Source: CAD feature listing. Evaluate the final solid. Frame: model axes, mm. Face numbers are marked on the shaded views. A direction names the side the tool comes from. Coordinates: 2 decimals unless noted, no trailing zeros. Write each loop counter-clockwise with the first axis right and the second up, starting at its lowest first coordinate (ties: lowest second). Pieces come first, ordered by that corner, then holes. Notation, with made-up numbers: (-13, 0.5) - (46, 0.5) arc R16 cw to (46, 24.5) - close; hole circle Ø3 at (72.25, 85.5). An arc over 180 degrees is marked (long way). One line per item, written item: value.
from build123d import *

# Parameters (mm, degrees)
SKETCH1_R           = 42.5
SKETCH1_R_2         = 12
BOSS_EXTRUDE1_DEPTH = 5
SKETCH2_R           = 32.5
SKETCH2_R_2         = 6.5
BOSS_EXTRUDE2_DEPTH = 10
SKETCH3_R           = 4
BOSS_EXTRUDE3_DEPTH = 10
SKETCH5_R           = 2.5
CUT_EXTRUDE1_DEPTH  = 10
SKETCH7_R           = 2.5
CUT_EXTRUDE2_DEPTH  = 10


with BuildPart() as part:
    # Sketch1 → Boss-Extrude1 (new body)
    with BuildSketch(Plane.XY):
        Circle(SKETCH1_R)
        Circle(SKETCH1_R_2, mode=Mode.SUBTRACT)
    extrude(amount=BOSS_EXTRUDE1_DEPTH)

    # Sketch2 → Boss-Extrude2 (add)
    with BuildSketch(Plane.XY.offset(5)):
        Circle(SKETCH2_R)
        Circle(SKETCH2_R_2, mode=Mode.SUBTRACT)
    extrude(amount=BOSS_EXTRUDE2_DEPTH)

    # Sketch3 → Boss-Extrude3 (add)
    with BuildSketch(Plane(origin=(0, 0, 0), x_dir=(-1, 0, 0), z_dir=(0, 0, -1))):
        with Locations(Location((0, 22.5, 0), (0, 0, 180))):
            Circle(SKETCH3_R)
        with Locations(Location((15.909902577, 15.909902577, 0), (0, 0, 180))):
            Circle(SKETCH3_R)
        with Locations(Location((22.5, 0, 0), (0, 0, 180))):
            Circle(SKETCH3_R)
        with Locations(Location((15.909902577, -15.909902577, 0), (0, 0, 180))):
            Circle(SKETCH3_R)
        with Locations(Location((0, -22.5, 0), (0, 0, 180))):
            Circle(SKETCH3_R)
        with Locations(Location((-15.909902577, -15.909902577, 0), (0, 0, 180))):
            Circle(SKETCH3_R)
        with Locations(Location((-22.5, 0, 0), (0, 0, 180))):
            Circle(SKETCH3_R)
        with Locations(Location((-15.909902577, 15.909902577, 0), (0, 0, 180))):
            Circle(SKETCH3_R)
    extrude(amount=BOSS_EXTRUDE3_DEPTH)

    # Sketch5 → Cut-Extrude1 (cut)
    with BuildSketch(Plane.XY.offset(15)):
        with Locations((0, 25)):
            Circle(SKETCH5_R)
        with Locations((21.650635095, 12.5)):
            Circle(SKETCH5_R)
        with Locations((21.650635095, -12.5)):
            Circle(SKETCH5_R)
        with Locations((0, -25)):
            Circle(SKETCH5_R)
        with Locations((-21.650635095, -12.5)):
            Circle(SKETCH5_R)
        with Locations((-21.650635095, 12.5)):
            Circle(SKETCH5_R)
    extrude(amount=-CUT_EXTRUDE1_DEPTH, mode=Mode.SUBTRACT)

    # Sketch7 → Cut-Extrude2 (cut)
    with BuildSketch(Plane.XY.offset(15)):
        with Locations((29, 0)):
            Circle(SKETCH7_R)
        with Locations((14.5, -25.11473671)):
            Circle(SKETCH7_R)
        with Locations((-14.5, -25.11473671)):
            Circle(SKETCH7_R)
        with Locations((-29, 0)):
            Circle(SKETCH7_R)
        with Locations((-14.5, 25.11473671)):
            Circle(SKETCH7_R)
        with Locations((14.5, 25.11473671)):
            Circle(SKETCH7_R)
    extrude(amount=-CUT_EXTRUDE2_DEPTH, mode=Mode.SUBTRACT)


solid = part.part
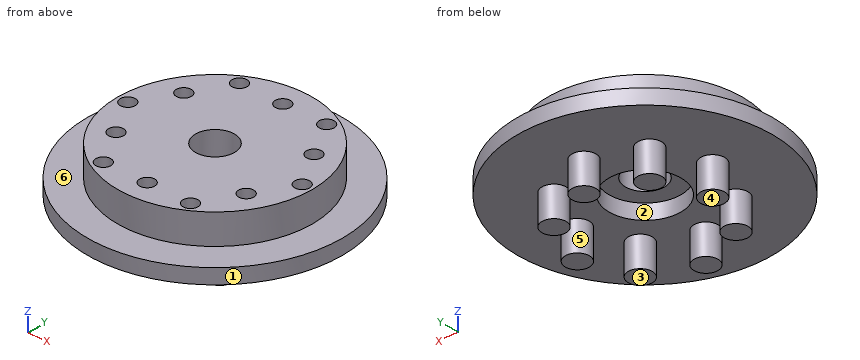
1) Material intervals for line 1 (Y direction, x = -14.5, z = 11.25); line 2 (Z direction, x = 6.5, y = -20); line 3 (Y direction, x = 0.5, z = 6.5), sorted ascending.
Values found:
line 1: -29.09 to -27.61, -22.61 to 22.61, 27.61 to 29.09
line 2: 0 to 15
line 3: -32.5 to -27.45, -22.55 to -6.48, 6.48 to 22.55, 27.45 to 32.5
2) Contact query for flat-ended pins moving along their axis: P1, Ø1.5, axis at x = -20, y = 7, coming from the -Z side; P2, Ø4, axis at y = -16.5, z = -7.5, coming from the -X side; P3, Ø12, axis at y = 32, z = -5.5, coming from the +X side; P4, Ø5, axis at x = 30, z = -7.5, coming from the -Y side. Output: stop coordinate, or through.
Values found:
P1: z = 0
P2: x = -19.91
P3: x = 30.5
P4: through
3) Reachability of the marked faces 4, 5 and 6 from +Z, -Z, +X, -X, +Y, -Y: full face, straight path, thin tool, end or side. Return the list, or none.
Values found:
face 4: -Z, +X, -X, +Y, -Y
face 5: -Z
face 6: +Z
4) Section query B-B on z = -5.25. Output: boundary loops of the cut face in (x, y).
Values found:
outline: circle Ø8 at (-22.5, 0); circle Ø8 at (-15.91, -15.91); circle Ø8 at (-15.91, 15.91); circle Ø8 at (0, -22.5); circle Ø8 at (0, 22.5); circle Ø8 at (15.91, -15.91); circle Ø8 at (15.91, 15.91); circle Ø8 at (22.5, 0)
5) Section query C-C on z = 7.5. State how many separate pieces and enclosed holes the cut face has, then the cut area to 3 significant figures.
Values found:
separate pieces: 1
enclosed holes: 13
area: 2,950 mm2
6) Draft query along Y for the marked faces 1, 2 and 3. Return one class per face: released by +Y, released by -Y, zero draft, split by the parting line, or undercut.
Values found:
face 1: split by the parting line
face 2: undercut
face 3: zero draft
7) Section query A-A on y = -5. Output: boundary loops of the cut face in (x, z).
Values found:
outline: (-42.2, 0) - (-10.91, 0) - (-10.91, 5) - (-4.15, 5) - (-4.15, 15) - (-32.11, 15) - (-32.11, 5) - (-42.2, 5) - close; (4.15, 5) - (10.91, 5) - (10.91, 0) - (42.2, 0) - (42.2, 5) - (32.11, 5) - (32.11, 15) - (4.15, 15) - close
8) Section query D-D on x = 10.5. Output: boundary loops of the cut face in (y, z), then the cut area to 3 significant figures.
Values found:
outline: (-41.18, 0) - (-5.81, 0) - (-5.81, 5) - (5.81, 5) - (5.81, 0) - (41.18, 0) - (41.18, 5) - (30.76, 5) - (30.76, 15) - (-30.76, 15) - (-30.76, 5) - (-41.18, 5) - close
area: 969 mm2
